from build123d import *

# Parameters (mm, degrees)
F0_R     = 4
F1_DEPTH = 5
F2_R     = 5.775
F2_R_2   = 4
F3_DEPTH = 4
F4_R     = 1.575
F5_DEPTH = 10
F6_SIZE  = 1
F7_SIZE  = 0.5
F8_R     = 0.2


with BuildPart() as f1:
    # F0 (on Front) → F1 (new body)
    with BuildSketch(Plane.XZ):
        Circle(F0_R)
    extrude(amount=F1_DEPTH)

    # F2 (on face) → F3 (join)
    with BuildSketch(Plane.XZ.offset(5)):
        Circle(F2_R)
        Circle(F2_R_2, mode=Mode.SUBTRACT)
        Circle(F2_R_2)
    extrude(amount=F3_DEPTH)

    # F4 (on face) → F5 (cut)
    with BuildSketch(Plane.XZ.offset(9)):
        Circle(F4_R)
    extrude(amount=-F5_DEPTH, mode=Mode.SUBTRACT)

    # F6
    f6_edges = [f1.edges().sort_by_distance(p)[0] for p in [
        (-5.775, -9, 0),
        (-5.775, -5, 0),
    ]]
    chamfer(f6_edges, length=F6_SIZE)

    # F7
    f7_edges = [f1.edges().sort_by_distance(p)[0] for p in [
        (-4, 0, 0),
    ]]
    chamfer(f7_edges, length=F7_SIZE)

    # F8
    f8_edges = [f1.edges().sort_by_distance(p)[0] for p in [
        (-1.575, -9, 0),
        (-1.575, 0, 0),
    ]]
    fillet(f8_edges, radius=F8_R)


solid = f1.part
Model file for the job. Use its own axes, mm. A direction names the side the tool comes from. Give positions to 0.01 mm unless a question says otherwise; leave off trailing zeros. Write each loop counter-clockwise with the first axis right and the second up, starting at its lowest first coordinate (ties: lowest second). Pieces come first, ordered by that corner, then holes. Notation, with made-up numbers: (17, 14) -> (21, 14) arc R23 cw to (21, 50) -> close; hole circle Ø9 at (24.5, 33). An arc over 180 degrees is marked (long way). Write item = value, one per line.
(1) Mould opens along X. For faces 3 (the face through (-0.867, -2.718, -3.905)), 4 (the face through (-1.25, -4.56, -0.96)), 5 (the face through (-2, 0, 1)) say: released by +X, released by -X, zero draft, split by the parting line, or undercut.
Determined:
face_3 = split by the parting line
face_4 = undercut
face_5 = zero draft
(2) Slice it at A-A, the plane x = 0. Give the cut face in (y, z) (3 decimals), then the cut area to 3 significant figures.
Determined:
outline = (-9, -4.775) -> (-8, -5.775) -> (-6, -5.775) -> (-5, -4.775) -> (-5, -4) -> (-0.5, -4) -> (0, -3.5) -> (0, -1.775) arc R0.2 ccw to (-0.2, -1.575) -> (-8.8, -1.575) arc R0.2 ccw to (-9, -1.775) -> close; (-9, 1.775) arc R0.2 ccw to (-8.8, 1.575) -> (-0.2, 1.575) arc R0.2 ccw to (0, 1.775) -> (0, 3.5) -> (-0.5, 4) -> (-5, 4) -> (-5, 4.775) -> (-6, 5.775) -> (-8, 5.775) -> (-9, 4.775) -> close
area = 55.6 mm2
(3) Flat gauge pins, fed straight in: P1, Ø3, axis at x = -2.5, z = 1, coming from the +Y side; P2, Ø2, axis at y = -5.5, z = -2.5, coming from the +X side; P3, Ø4, axis at y = -1, z = 0.5, coming from the -X side; P4, Ø3, axis at y = -2.5, z = -1, coming from the +X side. Where does each tip first touch, or does it go through?
Determined:
P1 = 0
P2 = 5.54
P3 = -4
P4 = 4
(4) Probe line 1 along Z through (x, y) = (-1, -3); line 2 along Z through (x, y) = (1.25, -1); line 3 along Y through (x, z) = (3, -2.75). List the from-to ranges inside material, lowest first.
Determined:
line_1 = -3.87 to -1.22, 1.22 to 3.87
line_2 = -3.8 to -0.96, 0.96 to 3.8
line_3 = -9 to -5
(5) Tool access for faces 1 (the face through (-1.25, -6.99, -5.64)), 2 (the face through (-3, -5, -3)): list every direction of +Z, -Z, +X, -X, +Y, -Y with a clear straight run to the whole face (end or side of a thin tool).
Determined:
face_1 = +Y, -Y
face_2 = +Y
(6) Slice it at B-B, the plane y = -3.75. Give the cut face in (x, z) (3 decimals).
Determined:
outline = circle Ø8 at (0, 0); hole circle Ø3.15 at (0, 0)
